Design review of the part built by this model. Coordinates are the model's own, in mm. Round coordinates to 2 decimals unless told otherwise and drop trailing zeros. Order: outer loops, then holes, each group sorted by start corner. A loop starts at its lowest first (then second) coordinate and runs counter-clockwise, first axis right, second up. Notation, with made-up numbers: M 7,62.5 L 18,62.5 A22 cw 18,72.5 Z; hole C 82.25,37.25 d3. An arc over 180 degrees is marked long. Write each question's results on one line, items separated by ' | '. Start each with the question number.
Item 1: Take a section at A-A, the plane x = -33.5. Write out the cut boundary in (y, z), plus the area to 3 significant figures.
Item 2: Wall thickness on line 1 (Y direction, x = -90.5, z = 1.05); line 2 (Y direction, x = -22, z = 1); line 3 (X direction, y = -14, z = -0.9): over which ranges is each line inside the solid? List them lowest first. Write a range as [from, to].
Item 3: Clearance check with flat-ended pins moving along their axes: pin 1 (2.5 mm diameter, centred on x = 140, y = -20, fed in from -Z); pin 2 (3.5 mm diameter, centred on x = 142.23, y = -77.45, fed in from -Z); pin 3 (3 mm diameter, centred on x = 8, z = -0.5, fed in from -Y); pin 4 (6.5 mm diameter, centred on x = -90, y = 42.7, fed in from -Z). State where each tip first meets the part, or that it passes through.
Item 4: Take a section at B-B, the plane y = 3. Write out the cut boundary in (x, z), plus the area to 3 significant figures.
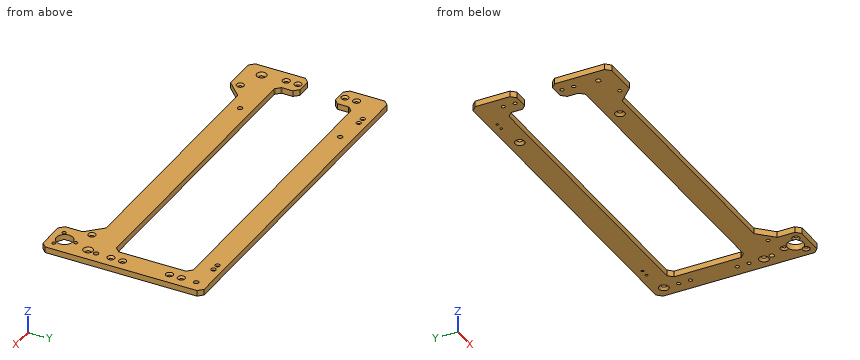
```python
from build123d import *

# Parameters (mm, degrees)
SKETCH_1_W          = 300
SKETCH_1_H          = 105.4
SKETCH_1_W_2        = 260
SKETCH_1_H_2        = 65.4
EXTRUDE_1_DEPTH     = 2.5
SKETCH_2_R          = 2.1
CUT_EXTRUDE_1_DEPTH = 160.066935596
SKETCH_3_R          = 1.6
CUT_EXTRUDE_2_DEPTH = 160.066935596
CHAMFER_1_SIZE      = 1.5
CHAMFER_2_SIZE      = 2
SKETCH_5_W          = 20
SKETCH_5_H          = 30
CUT_EXTRUDE_5_DEPTH = 160.066935596
EXTRUDE_2_DEPTH     = 5
SKETCH_7_R          = 1.6
SKETCH_7_R_2        = 2.1
CUT_EXTRUDE_6_DEPTH = 164.833726687
CHAMFER_4_SIZE      = 2
CHAMFER_5_SIZE      = 1.5
SKETCH_8_W          = 32
SKETCH_8_H          = 19
EXTRUDE_3_DEPTH     = 5
CHAMFER_3_SIZE      = 4
FILLET_1_R          = 1
SKETCH_9_R          = 7
SKETCH_9_R_2        = 1.6
CUT_EXTRUDE_7_DEPTH = 173.334239198
CHAMFER_6_SIZE      = 1.5
SKETCH_10_R         = 1.05
CUT_EXTRUDE_8_DEPTH = 173.334239201
CHAMFER_7_SIZE      = 1


with BuildPart() as part:
    # 草图1 → 凸台-拉伸1 (new, symmetric)
    with BuildSketch(Plane.XY):
        Rectangle(SKETCH_1_W, SKETCH_1_H)
        Rectangle(SKETCH_1_W_2, SKETCH_1_H_2, mode=Mode.SUBTRACT)
    extrude(amount=EXTRUDE_1_DEPTH, both=True)

    # 草图2 → 切除-拉伸1 (cut, through all)
    with BuildSketch(Plane.XY.offset(2.5)):
        with Locations((-90, 42.7)):
            Circle(SKETCH_2_R)
        with Locations((140, 42.7)):
            Circle(SKETCH_2_R)
        with Locations((-90, -42.7)):
            Circle(SKETCH_2_R)
        with Locations((140, -42.7)):
            Circle(SKETCH_2_R)
    extrude(amount=-CUT_EXTRUDE_1_DEPTH, mode=Mode.SUBTRACT)

    # 草图3 → 切除-拉伸2 (cut, through all)
    with BuildSketch(Plane.XY.offset(2.5)):
        with Locations((140, 30)):
            Circle(SKETCH_3_R)
        with Locations((140, -30)):
            Circle(SKETCH_3_R)
        with Locations((140, 20)):
            Circle(SKETCH_3_R)
        with Locations((140, -20)):
            Circle(SKETCH_3_R)
        with Locations(Location((-140, -30, 0), (0, 0, 180))):
            Circle(SKETCH_3_R)
        with Locations(Location((-140, -20, 0), (0, 0, 180))):
            Circle(SKETCH_3_R)
        with Locations(Location((-140, 20, 0), (0, 0, 180))):
            Circle(SKETCH_3_R)
        with Locations(Location((-140, 30, 0), (0, 0, 180))):
            Circle(SKETCH_3_R)
    extrude(amount=-CUT_EXTRUDE_2_DEPTH, mode=Mode.SUBTRACT)

    # 倒角1
    chamfer_1_edges = [part.edges().sort_by_distance(p)[0] for p in [
        (-138.4, -30, 2.5),
        (138.4, -20, 2.5),
        (138.4, 20, 2.5),
        (138.4, -30, 2.5),
        (-138.4, -20, 2.5),
        (-138.4, 20, 2.5),
        (-138.4, 30, 2.5),
        (138.4, 30, 2.5),
    ]]
    chamfer(chamfer_1_edges, length=CHAMFER_1_SIZE)

    # 倒角2
    chamfer_2_edges = [part.edges().sort_by_distance(p)[0] for p in [
        (137.9, 42.7, -2.5),
        (-92.1, -42.7, -2.5),
        (137.9, -42.7, -2.5),
        (-92.1, 42.7, -2.5),
    ]]
    chamfer(chamfer_2_edges, length=CHAMFER_2_SIZE)

    # 草图5 → 切除-拉伸5 (cut, through all)
    with BuildSketch(Plane(origin=(0, 0, -2.5), x_dir=(-1, 0, 0), z_dir=(0, 0, -1))):
        with Locations((140, 0)):
            Rectangle(SKETCH_5_W, SKETCH_5_H)
    extrude(amount=-CUT_EXTRUDE_5_DEPTH, mode=Mode.SUBTRACT)

    # 草图6 → 凸台-拉伸2 (add)
    with BuildSketch(Plane(origin=(0, 0, -2.5), x_dir=(-1, 0, 0), z_dir=(0, 0, -1))):
        Polygon((150, -52.7), (150, -65.7), (118, -65.7), (105, -52.7), align=None)
        Polygon((-118, -65.7), (-105, -52.7), (-150, -52.7), (-150, -65.7), align=None)
    extrude(amount=-EXTRUDE_2_DEPTH)

    # 草图7 → 切除-拉伸6 (cut, through all)
    with BuildSketch(Plane(origin=(0, 0, -2.5), x_dir=(-1, 0, 0), z_dir=(0, 0, -1))):
        with Locations((118.485281374, -57.7)):
            Circle(SKETCH_7_R)
        with Locations((-118.485281374, -57.7)):
            Circle(SKETCH_7_R)
        with Locations((138.5, -50.2)):
            Circle(SKETCH_7_R_2)
        with Locations(Location((-138.5, -50.2, 0), (0, 0, 180))):
            Circle(SKETCH_7_R_2)
    extrude(amount=-CUT_EXTRUDE_6_DEPTH, mode=Mode.SUBTRACT)

    # 倒角4
    chamfer_4_edges = [part.edges().sort_by_distance(p)[0] for p in [
        (136.4, -50.2, 2.5),
        (-136.4, -50.2, 2.5),
    ]]
    chamfer(chamfer_4_edges, length=CHAMFER_4_SIZE)

    # 倒角5
    chamfer_5_edges = [part.edges().sort_by_distance(p)[0] for p in [
        (120.085281374, -57.7, 2.5),
        (-116.885281374, -57.7, 2.5),
    ]]
    chamfer(chamfer_5_edges, length=CHAMFER_5_SIZE)

    # 草图8 → 凸台-拉伸3 (add)
    with BuildSketch(Plane.XY.offset(2.5)):
        with Locations((134, -75.2)):
            Rectangle(SKETCH_8_W, SKETCH_8_H)
    extrude(amount=-EXTRUDE_3_DEPTH)

    # 倒角3
    chamfer_3_edges = [part.edges().sort_by_distance(p)[0] for p in [
        (-130, -15, 0),
        (-130, 15, 0),
        (-150, 15, 0),
        (-150, -15, 0),
        (-150, -65.7, 0),
        (-130, 32.7, 0),
        (-130, -32.7, 0),
        (130, -32.7, 0),
        (130, 32.7, 0),
        (150, -84.7, 0),
        (118, -84.7, 0),
        (-150, 52.7, 0),
        (150, 52.7, 0),
    ]]
    chamfer(chamfer_3_edges, length=CHAMFER_3_SIZE)

    # 圆角1
    fillet_1_edges = [part.edges().sort_by_distance(p)[0] for p in [
        (-105, -52.7, 0),
        (105, -52.7, 0),
        (118, -65.7, 0),
        (-130, 28.7, 0),
        (-130, -28.7, 0),
        (126, -32.7, 0),
        (-126, -32.7, 0),
        (126, 32.7, 0),
        (-126, 32.7, 0),
        (130, -28.7, 0),
        (130, 28.7, 0),
    ]]
    fillet(fillet_1_edges, radius=FILLET_1_R)

    # 草图9 → 切除-拉伸7 (cut, through all)
    with BuildSketch(Plane.XY.offset(2.5)):
        with Locations((134, -72.7)):
            Circle(SKETCH_9_R)
        with Locations((134, -63.2)):
            Circle(SKETCH_9_R_2)
        with Locations((142.227241336, -77.45)):
            Circle(SKETCH_9_R_2)
        with Locations((125.772758664, -77.45)):
            Circle(SKETCH_9_R_2)
    extrude(amount=-CUT_EXTRUDE_7_DEPTH, mode=Mode.SUBTRACT)

    # 倒角6
    # the kernel refuses this chamfer: 1.5 mm, written as the material it takes off along each edge
    with BuildSketch(Plane(origin=(125.772758664, -77.45, -2.5), x_dir=(1, 0, 0), z_dir=(0, -1, 0))) as chamfer_6_piece_1:
        Polygon((1.6, CHAMFER_6_SIZE), (1.6 + CHAMFER_6_SIZE, 0), (1.6, 0), align=None)
    revolve(axis=Axis((125.772758664, -77.45, -2.5), (0, 0, 1)), mode=Mode.SUBTRACT)
    with BuildSketch(Plane(origin=(142.227241336, -77.45, -2.5), x_dir=(1, 0, 0), z_dir=(0, -1, 0))) as chamfer_6_piece_2:
        Polygon((1.6, CHAMFER_6_SIZE), (1.6 + CHAMFER_6_SIZE, 0), (1.6, 0), align=None)
    revolve(axis=Axis((142.227241336, -77.45, -2.5), (0, 0, 1)), mode=Mode.SUBTRACT)
    with BuildSketch(Plane(origin=(134, -63.2, -2.5), x_dir=(1, 0, 0), z_dir=(0, -1, 0))) as chamfer_6_piece_3:
        Polygon((1.6, CHAMFER_6_SIZE), (1.6 + CHAMFER_6_SIZE, 0), (1.6, 0), align=None)
    revolve(axis=Axis((134, -63.2, -2.5), (0, 0, 1)), mode=Mode.SUBTRACT)

    # 草图10 → 切除-拉伸8 (cut, through all)
    with BuildSketch(Plane(origin=(0, 0, -2.5), x_dir=(-1, 0, 0), z_dir=(0, 0, -1))):
        with Locations((120.223206297, 45.8)):
            Circle(SKETCH_10_R)
        with Locations((113.723206297, 45.8)):
            Circle(SKETCH_10_R)
        with Locations(Location((-111.723206297, 45.8, 0), (0, 0, 180))):
            Circle(SKETCH_10_R)
        with Locations(Location((-118.223206297, 45.8, 0), (0, 0, 180))):
            Circle(SKETCH_10_R)
    extrude(amount=-CUT_EXTRUDE_8_DEPTH, mode=Mode.SUBTRACT)

    # 倒角7
    chamfer_7_edges = [part.edges().sort_by_distance(p)[0] for p in [
        (-119.173206297, 45.8, 2.5),
        (-112.673206297, 45.8, 2.5),
        (110.673206297, 45.8, 2.5),
        (117.173206297, 45.8, 2.5),
    ]]
    chamfer(chamfer_7_edges, length=CHAMFER_7_SIZE)


solid = part.part
```
Results list:
1) outline: M -52.7,-2.5 L -32.7,-2.5 L -32.7,2.5 L -52.7,2.5 Z; M 32.7,-2.5 L 52.7,-2.5 L 52.7,2.5 L 32.7,2.5 Z | area: 200 mm²
2) line 1: [-52.7, -44.74], [-40.66, -32.7], [32.7, 40.66], [44.74, 52.7] | line 2: [-52.7, -32.7], [32.7, 52.7] | line 3: [130, 150]
3) pin 1: through | pin 2: z = -1.15 | pin 3: y = -52.7 | pin 4: z = -1.65
4) outline: M 130,-2.5 L 150,-2.5 L 150,2.5 L 130,2.5 Z | area: 100 mm²
